Read the model definition and answer for the solid it produces. Units are mm, in the model's axes. Face numbers are marked on the shaded views. Give positions to 0.01 mm unless a question says otherwise; leave off trailing zeros. Order: outer loops, then holes, each group sorted by start corner. A loop starts at its lowest first (then second) coordinate and runs counter-clockwise, first axis right, second up. Notation, with made-up numbers: (13.5, 27.5) -> (58.5, 27.5) arc R18 cw to (58.5, 34.5) -> close; hole circle Ø8 at (59.25, -12.75). An arc over 180 degrees is marked (long way). Answer as CSV lines item,"result". Start each with the question number.
1) Find section C-C (z = 60). Determine the outline of the cut face in (x, y).
2) Find section A-A (y = -25.5). Determine the outline of the cut face in (x, z) (3 decimals), and give its area (3 significant figures).
3) Find section D-D (z = -59). Determine the outline of the cut face in (x, y), and give its area (3 significant figures).
4) Find section B-B (x = -69). Determine the outline of the cut face in (y, z).
5) The mould has two halves that part along Z. Classify the marked faces 1, 2 and 3: +Z half, -Z half, draft (parallel to the pull), parting line (faces both ways), or undercut.
6) Flat-ended cylindrical pins translate along their axes: pin 1 Ø6 at (x, y) = (17.5, -54) entering from -Z; pin 2 Ø9.5 at (x, z) = (28, 105) entering from +Y; pin 3 Ø3.5 at (x, z) = (-130.77, -71.89) entering from -Y; pin 4 Ø2 at (x, y) = (100, -48.5) entering from +Z. Find the tip coordinate at first contact, or state that the pin passes through.
7) Straight lines are drawn through the part: L1, parallel to Z at x = -57, y = -61.5; L2, parallel to Z at x = -116, y = -61; L3, parallel to Z at x = 14.5, y = -35. For each, find the intervals that lie inside material, in ascending order. Write a range as from..to.
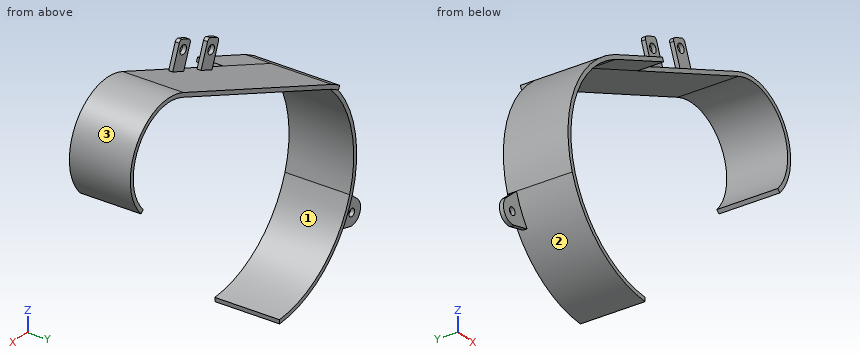
```python
from build123d import *

# Parameters (mm, degrees)
BASE_FLANGE2_DEPTH  = 63.5
SKETCH8_W           = 331.965977541
SKETCH8_H           = 30.9372
CUT_EXTRUDE1_DEPTH  = 256.834789278
SKETCH9_W           = 150.054784792
SKETCH9_H           = 34.679027416
CUT_EXTRUDE2_DEPTH  = 256.834789278
BOSS_EXTRUDE1_DEPTH = 20.32
SKETCH12_W          = 12.7
SKETCH12_H          = 3.175
BOSS_EXTRUDE2_DEPTH = 21.59
SKETCH13_R          = 3.5
CUT_EXTRUDE5_DEPTH  = 21.59
FILLET1_R           = 2.54
SKETCH14_R          = 3
BOSS_EXTRUDE3_DEPTH = 3.175


# Sheet-metal steps are written as plain solids
with BuildPart() as part:
    # Sketch1 → Base-Flange2 (new body)
    with BuildSketch(Plane(origin=(0, 0, 0), x_dir=(1, 0, 0), z_dir=(0, 1, 0))):
        with BuildLine():
            Line((80.769724328, -109.524319493), (-79.196155859, -46.179527064))
            ThreePointArc((-79.196155859, -46.179527064), (-120.807882744, -4.431069312), (-123.261655777, 54.4624663))
            ThreePointArc((-123.261655777, 54.4624663), (-94.143629301, 94.693559024), (-47.619751411, 112.069665426))
            Line((-47.619751411, 112.069665426), (-47.822872467, 115.238161415))
            ThreePointArc((-47.822872467, 115.238161415), (-96.069602275, 97.217694761), (-126.264058949, 55.495051727))
            ThreePointArc((-126.264058949, 55.495051727), (-123.704959468, -5.730431564), (-80.422032808, -49.108963745))
            Line((-80.422032808, -49.108963745), (79.600772216, -112.476297806))
            ThreePointArc((79.600772216, -112.476297806), (129.785334621, -96.938999369), (125.376413714, -44.589602401))
            Line((125.376413714, -44.589602401), (123.077927873, -46.779942064))
            ThreePointArc((123.077927873, -46.779942064), (127.152879464, -95.163948708), (80.769724328, -109.524319493))
        make_face()
    extrude(amount=-BASE_FLANGE2_DEPTH)

    # Sketch8 → Cut-Extrude1 (cut, through all)
    with BuildSketch(Plane(origin=(-27.711967852, 0, 69.98159058), x_dir=(0.9297569489485495, 0, 0.36817389353657926), z_dir=(-0.36817389353657926, 0, 0.9297569489485495))):
        with Locations((13.838804259, 0)):
            Rectangle(SKETCH8_W, SKETCH8_H)
    extrude(amount=-CUT_EXTRUDE1_DEPTH, mode=Mode.SUBTRACT)

    # Sketch9 → Cut-Extrude2 (cut, through all)
    with BuildSketch(Plane(origin=(-27.711967852, 0, 69.98159058), x_dir=(0.9297569489485495, 0, 0.36817389353657926), z_dir=(-0.36817389353657926, 0, 0.9297569489485495))):
        with Locations((-140.963680017, -15.4686)):
            Rectangle(SKETCH9_W, SKETCH9_H)
    extrude(amount=-CUT_EXTRUDE2_DEPTH, mode=Mode.SUBTRACT)

    # Sketch11 → Boss-Extrude1 (add)
    with BuildSketch(Plane.XZ.offset(63.5)):
        with BuildLine():
            Line((-47.619751411, -112.069665426), (-47.822872467, -115.238161415))
            ThreePointArc((-47.822872467, -115.238161415), (-96.069602275, -97.217694761), (-126.264058949, -55.495051727))
            ThreePointArc((-126.264058949, -55.495051727), (-123.704959468, 5.730431564), (-80.422032808, 49.108963745))
            Line((-80.422032808, 49.108963745), (-29.009735812, 69.467688228))
            Line((-29.009735812, 69.467688228), (-27.8407837, 66.515709916))
            Line((-27.8407837, 66.515709916), (-79.196155859, 46.179527064))
            ThreePointArc((-79.196155859, 46.179527064), (-120.807882744, 4.431069312), (-123.261655777, -54.4624663))
            ThreePointArc((-123.261655777, -54.4624663), (-94.143629301, -94.693559024), (-47.619751411, -112.069665426))
        make_face()
    extrude(amount=BOSS_EXTRUDE1_DEPTH)

    # Sketch12 → Boss-Extrude2 (add)
    with BuildSketch(Plane(origin=(-27.711967852, 0, 69.98159058), x_dir=(0.9297569489485495, 0, 0.3681738935365793), z_dir=(-0.36817389353657937, 0, 0.9297569489485495))):
        with Locations((27.459636868, -58.7121)):
            Rectangle(SKETCH12_W, SKETCH12_H)
        with Locations((60.299587615, -58.7121)):
            Rectangle(SKETCH12_W, SKETCH12_H)
    extrude(amount=BOSS_EXTRUDE2_DEPTH)

    # Sketch13 → Cut-Extrude5 (cut)
    with BuildSketch(Plane(origin=(0, -57.1246, 0), x_dir=(1, 0, 0), z_dir=(0, 1, 0))):
        with Locations(Location((22.976705445, -105.756645834, 0), (0, 0, 270))):
            Circle(SKETCH13_R)
        with Locations(Location((-7.181091285, -92.717889538, 0), (0, 0, 270))):
            Circle(SKETCH13_R)
    extrude(amount=-CUT_EXTRUDE5_DEPTH, mode=Mode.SUBTRACT)

    # Fillet1
    fillet1_edges = [part.edges().sort_by_distance(p)[0] for p in [
        (-4.226097394, -58.7121, 102.502868753),
        (-16.034010646, -58.7121, 97.827060305),
        (26.307075016, -58.7121, 114.593681283),
        (14.499161765, -58.7121, 109.917872835),
    ]]
    fillet(fillet1_edges, radius=FILLET1_R)

    # Sketch14 → Boss-Extrude3 (add)
    with BuildSketch(Plane(origin=(0, -36.672703388, 0), x_dir=(1, 0, 0), z_dir=(0, 1, 0))):
        with BuildLine():
            Line((-136.967303974, 64.658320793), (-126.264058949, 55.495051727))
            ThreePointArc((-126.264058949, 55.495051727), (-121.330527713, 67.047255445), (-114.82018179, 77.790091998))
            Line((-114.82018179, 77.790091998), (-128.504840161, 81.144951055))
            ThreePointArc((-128.504840161, 81.144951055), (-139.246667683, 76.243475882), (-136.967303974, 64.658320793))
        make_face()
        with Locations(Location((-130.77278095, 71.8938933, 0), (0, 0, 270))):
            Circle(SKETCH14_R, mode=Mode.SUBTRACT)
    extrude(amount=-BOSS_EXTRUDE3_DEPTH)


solid = part.part
```
Findings below:
1,outline,"(-52.92, -83.82) -> (-44.3, -83.82) -> (-44.3, -15.47) -> (-52.92, -15.47) -> close; (131.34, -63.5) -> (134.71, -63.5) -> (134.71, -15.47) -> (131.34, -15.47) -> close"
2,outline,"(-88.699, 44.902) -> (-87.516, 41.916) arc R81.28 cw to (-79.196, 46.18) -> (80.77, 109.524) arc R38.74 cw to (123.078, 46.78) -> (125.376, 44.59) arc R41.915 ccw to (79.601, 112.476) -> (-80.422, 49.109) arc R84.455 ccw to start"
2,area,"923 mm²"
3,outline,"(-130.36, -39.85) -> (-124.97, -39.85) -> (-124.97, -83.82) -> (-121.55, -83.82) -> (-121.55, -32.81) -> (-124.97, -32.81) -> (-124.97, -36.67) -> (-130.36, -36.67) -> close"
3,area,"192 mm²"
4,outline,"(-83.82, -111.27) -> (-32.81, -111.27) -> (-32.81, -107.93) -> (-83.82, -107.93) -> close; (-83.82, 50.22) -> (-15.47, 50.22) -> (-15.47, 53.63) -> (-83.82, 53.63) -> close"
5,face 1,"undercut"
5,face 2,"-Z half"
5,face 3,"parting line"
6,pin 1,"z = 83.28"
6,pin 2,"y = -57.12"
6,pin 3,"through"
6,pin 4,"z = 115.23"
7,L1,"-114.17..-110.95, 54.97..58.38"
7,L2,"-76.08..-70.14, 13.73..19.6"
7,L3,"83.28..86.7"
